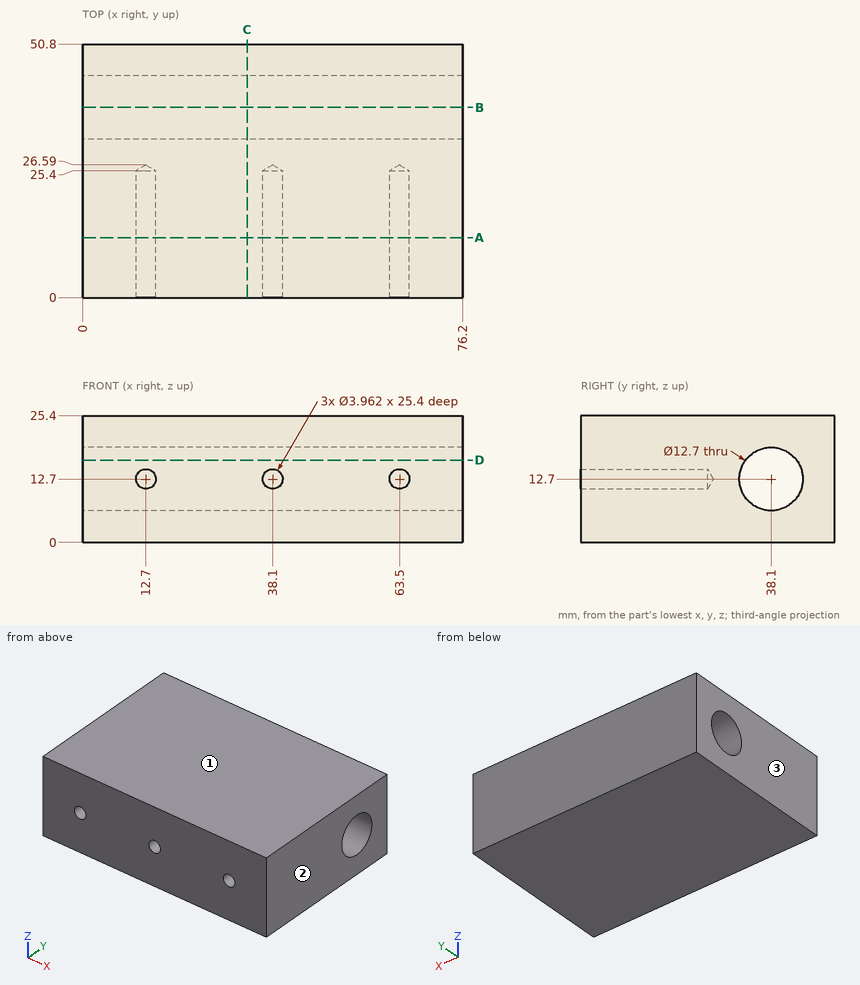
The drawing under review shows one solid part. Ordinate dimensions are in mm from its lowest x, y, z. Round coordinates to 2 decimals unless told otherwise and drop trailing zeros. Order: outer loops, then holes, each group sorted by start corner. A loop starts at its lowest first (then second) coordinate and runs counter-clockwise, first axis right, second up. Notation, with made-up numbers: (-25, 17) -> (-12, 17) arc R15 cw to (-12, 25) -> close; hole circle Ø3 at (82.25, -7.75). An arc over 180 degrees is marked (long way). Return JSON: item names as keys, results as strings.
1. Take a section at C-C (x = 33). Write out the cut boundary in (y, z), then the cut area to 3 significant figures.
Answer block:
{"outline": "(0, 0) -> (50.8, 0) -> (50.8, 25.4) -> (0, 25.4) -> close; hole circle Ø12.7 at (38.1, 12.7)", "area": "1,160 mm²"}
2. Take a section at A-A (y = 12). Write out the cut boundary in (x, z), then the cut area to 3 significant figures.
Answer block:
{"outline": "(0, 0) -> (76.2, 0) -> (76.2, 25.4) -> (0, 25.4) -> close; hole circle Ø3.96 at (12.7, 12.7); hole circle Ø3.96 at (38.1, 12.7); hole circle Ø3.96 at (63.5, 12.7)", "area": "1,900 mm²"}
3. For L1, parallel to X at y = 18, z = 12.7; L2, parallel to Z at x = 37, y = 38; L3, parallel to Y at x = 45.5, z = 12.7, list the stretches that pass through material, from the lowest coordinate up. Write a range as [from, to].
Answer block:
{"L1": "x = [0, 10.72], [14.68, 36.12], [40.08, 61.52], [65.48, 76.2]", "L2": "z = [0, 6.35], [19.05, 25.4]", "L3": "y = [0, 31.75], [44.45, 50.8]"}
4. Take a section at D-D (z = 16.5). Write out the cut boundary in (x, y), then the cut area to 3 significant figures.
Answer block:
{"outline": "(0, 0) -> (76.2, 0) -> (76.2, 33.01) -> (0, 33.01) -> close; (0, 43.19) -> (76.2, 43.19) -> (76.2, 50.8) -> (0, 50.8) -> close", "area": "3,100 mm²"}
5. Take a section at B-B (y = 38.1). Write out the cut boundary in (x, z).
Answer block:
{"outline": "(0, 0) -> (76.2, 0) -> (76.2, 6.35) -> (0, 6.35) -> close; (0, 19.05) -> (76.2, 19.05) -> (76.2, 25.4) -> (0, 25.4) -> close"}
6. Insertion check: P1, Ø3, axis at y = 36, z = 9, coming from the +X side. The pin has a flat end and moves straight along its axis. Give the tip position at first contact, or say it passes through.
Answer block:
{"P1": "passes through"}
7. The part is to be moulded in two halves that separate along X. For the marked faces 1, 2 and 3, say which applies: +X half, -X half, draft (parallel to the pull), parting line (faces both ways), or undercut.
Answer block:
{"face 1": "draft", "face 2": "+X half", "face 3": "-X half"}
